Verification items for the finished model (mm, model axes). Face numbers are marked on the shaded views. A direction names the side the tool comes from. Coordinates: 2 decimals unless noted, no trailing zeros. Order: outer loops, then holes, each group sorted by start corner. A loop starts at its lowest first (then second) coordinate and runs counter-clockwise, first axis right, second up. Notation, with made-up numbers: (13.5, 5) -> (22.5, 5) arc R16 ccw to (22.5, 26) -> close; hole circle Ø7 at (69, -11). An arc over 180 degrees is marked (long way). Answer as CSV lines item,"result".
```python
from build123d import *

# Parameters (mm, degrees)
SKETCH001_W     = 6.5
SKETCH001_H     = 6.5
POCKET_DEPTH    = 10
POCKET001_DEPTH = 40


with BuildPart() as part:
    # Sketch → Revolution (revolve)
    with BuildSketch(Plane.XZ):
        Polygon((0, 0), (-11.635, 0), (-11.635, 40), (-8.125, 50), (-8.125, 60), (0, 60), (0, 50), (-4.5, 50), (-4.5, 40), (0, 40), align=None)
    revolve(axis=Axis((0, 0, 0), (0, 0, 1)))

    # Sketch001 (on DatumPlane) → Pocket (cut)
    with BuildSketch(Plane.XY.offset(60)):
        Rectangle(SKETCH001_W, SKETCH001_H)
    extrude(amount=-POCKET_DEPTH, mode=Mode.SUBTRACT)

    # Sketch002 → Pocket001 (cut)
    with BuildSketch(Plane.XY):
        Polygon((10.33457, 0), (5.167285, 8.95), (-5.167285, 8.95), (-10.33457, 0), (-5.167285, -8.95), (5.167285, -8.95), align=None)
    extrude(amount=POCKET001_DEPTH, mode=Mode.SUBTRACT)


solid = part.part
```
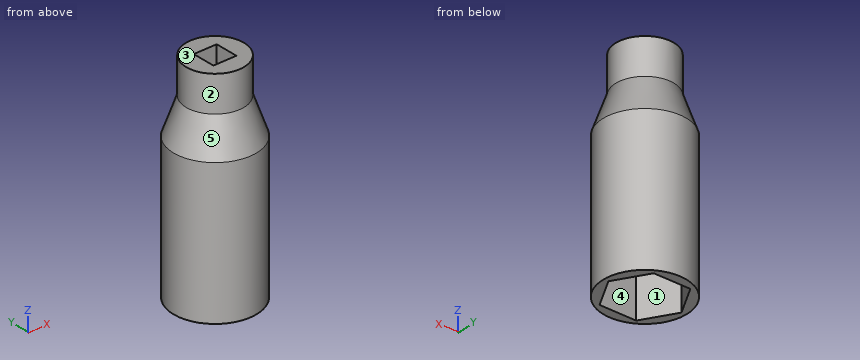
Item 1: Release check for a two-part mould opening along Y. For the marked faces 1, 2 and 3 record: +Y half, -Y half, draft (parallel to the pull), parting line (faces both ways), or undercut.
Answer list:
face 1,"undercut"
face 2,"parting line"
face 3,"draft"
Item 2: Thickness scan on line 1 (Z direction, x = -3, y = -3.75); line 2 (Y direction, x = 9.75, z = 10); line 3 (X direction, y = -3.25, z = 32.5). Record the ranges inside material, lowest first.
Answer list:
line 1,"40 to 60"
line 2,"-6.35 to -1.01, 1.01 to 6.35"
line 3,"-11.17 to -8.46, 8.46 to 11.17"
Item 3: Section check C-C, the plane z = 52. Record the boundary of the cut face in (x, y) (3 decimals), plus the area to 3 significant figures.
Answer list:
outline,"circle Ø16.25 at (0, 0); hole (-3.25, -3.25) -> (3.25, -3.25) -> (3.25, 3.25) -> (-3.25, 3.25) -> close"
area,"165 mm2"
Item 4: Depth check by flat-ended pin: pin 1 Ø2 at (y, z) = (-1.5, 24.5) entering from +X; pin 2 Ø4 at (y, z) = (6.5, 21.5) entering from -X; pin 3 Ø0.6 at (x, y) = (3.5, 1) entering from -Z. Enter the tip coordinate at first touch or a pass-through.
Answer list:
pin 1,"x = 11.62"
pin 2,"x = -10.73"
pin 3,"z = 50"
Item 5: Tool access check on the marked faces 4 and 5. Record the directions out of +Z, -Z, +X, -X, +Y, -Y that give a thin tool (end or side, any length) a straight path to the whole face; none if there is none.
Answer list:
face 4,"-Z"
face 5,"+Z"
Item 6: Section check A-A, the plane x = 0. Record the boundary of the cut face in (y, z) (3 decimals), plus the area to 3 significant figures.
Answer list:
outline,"(-11.635, 0) -> (-8.95, 0) -> (-8.95, 40) -> (-4.5, 40) -> (-4.5, 50) -> (-3.25, 50) -> (-3.25, 60) -> (-8.125, 60) -> (-8.125, 50) -> (-11.635, 40) -> close; (3.25, 50) -> (4.5, 50) -> (4.5, 40) -> (8.95, 40) -> (8.95, 0) -> (11.635, 0) -> (11.635, 40) -> (8.125, 50) -> (8.125, 60) -> (3.25, 60) -> close"
area,"420 mm2"
Item 7: Section check B-B, the plane z = 10. Record the boundary of the cut face in (x, y) (3 decimals).
Answer list:
outline,"circle Ø23.27 at (0, 0); hole (-10.335, 0) -> (-5.167, -8.95) -> (5.167, -8.95) -> (10.335, 0) -> (5.167, 8.95) -> (-5.167, 8.95) -> close"
